Geometry: final body of the model. Coordinates: model frame, mm. Give positions to 0.01 mm unless a question says otherwise; leave off trailing zeros. Loops run counter-clockwise (first coordinate to the right, second up) from the corner with the lowest first, then second, coordinate; pieces in that order, holes last. Notation, with made-up numbers: (45.25, -13) - (88.25, -13) arc R12 cw to (88.25, 1) - close; hole circle Ø5 at (-38.75, 58). An arc over 180 degrees is marked (long way). Answer in a Markdown table with one row per item.
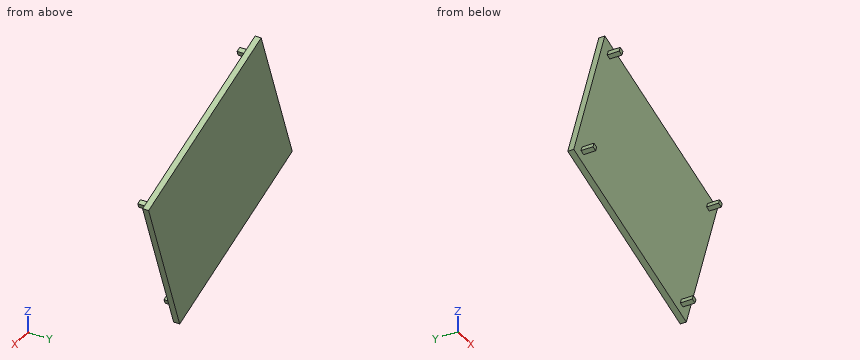
from build123d import *

# Parameters (mm, degrees)
EXTRUDE_1_DEPTH = 5
EXTRUDE_2_DEPTH = 10


with BuildPart() as part:
    # 草图2 → 凸台-拉伸1 (new body)
    with BuildSketch(Plane(origin=(0, 0, 0), x_dir=(1, 0, 0), z_dir=(0, 1, 0))):
        Polygon((-101.961949946, 31.82244298), (57.849497127, 89.790549593), (101.961949946, -31.82244298), (-57.849497127, -89.790549593), align=None)
    extrude(amount=EXTRUDE_1_DEPTH)

    # 草图3 → 凸台-拉伸2 (add)
    with BuildSketch(Plane(origin=(0, 0, 0), x_dir=(1, 0, 0), z_dir=(0, 1, 0))):
        Polygon((-53.056842775, -79.542085251), (-49.296573432, -78.178129801), (-50.760983059, -74.140919768), (-54.521252402, -75.504875218), align=None)
        Polygon((87.953231018, -28.393770643), (91.713500361, -27.029815193), (90.364794207, -23.311586416), (86.604524864, -24.675541865), align=None)
        Polygon((50.660555447, 74.417875215), (54.42082479, 75.781830665), (53.058052487, 79.538838208), (49.297783144, 78.174882759), align=None)
        Polygon((-90.349544911, 23.26954585), (-86.589275569, 24.6335013), (-87.969378224, 28.438286645), (-91.729647567, 27.074331195), align=None)
    extrude(amount=-EXTRUDE_2_DEPTH)


solid = part.part
Q1. Cut plane B-B (x = -42.5). Output: boundary loops of the cut face in (y, z).
Check values:
| item | result |
|---|---|
| outline | (0, -53.39) - (5, -53.39) - (5, 84.22) - (0, 84.22) - close |
Q2. Material intervals for line 1 along Y through (x, z) = (67, -4.5); line 2 along Z through (x, y) = (45, 3); line 3 along Z through (x, y) = (-52.5, -8.5), sorted ascending.
Check values:
| item | result |
|---|---|
| line 1 | 0 to 5 |
| line 2 | -85.13 to 52.48 |
| line 3 | 74.77 to 79.34 |
Q3. Cut plane C-C (z = -50.5). Output: boundary loops of the cut face in (x, y).
Check values:
| item | result |
|---|---|
| outline | (-50.47, 0) - (72.1, 0) - (72.1, 5) - (-50.47, 5) - close |
Q4. Cut plane A-A (y = -3.75). Output: boundary loops of the cut face in (x, z).
Check values:
| item | result |
|---|---|
| outline | (-91.73, -27.07) - (-87.97, -28.44) - (-86.59, -24.63) - (-90.35, -23.27) - close; (-54.52, 75.5) - (-50.76, 74.14) - (-49.3, 78.18) - (-53.06, 79.54) - close; (49.3, -78.17) - (53.06, -79.54) - (54.42, -75.78) - (50.66, -74.42) - close; (86.6, 24.68) - (90.36, 23.31) - (91.71, 27.03) - (87.95, 28.39) - close |
Q5. First-contact query: pin 1 (2 mm diameter, centred on x = -54.5, z = 41.5, fed in from -Y); pin 2 (2 mm diameter, centred on x = -22, y = 2.5, fed in from +Z). Flat tips, straight axial feed; report the tip coordinate or a pass-through.
Check values:
| item | result |
|---|---|
| pin 1 | y = 0 |
| pin 2 | z = 77.15 |
